from build123d import *

# Parameters (mm, degrees)
SKETCH2_R                = 6.25
BOSS_EXTRUDE1_DEPTH      = 24
BOSS_EXTRUDE1_DEPTH_BACK = 24
BOSS_EXTRUDE2_START      = 1
BOSS_EXTRUDE2_DEPTH      = 12.5
SKETCH5_R                = 5
BOSS_EXTRUDE4_DEPTH      = 10
BOSS_EXTRUDE4_DEPTH_BACK = 54
SKETCH6_R                = 6
BOSS_EXTRUDE5_DEPTH      = 31
BOSS_EXTRUDE5_DEPTH_BACK = 30


with BuildPart() as part:
    # Sketch2 → Boss-Extrude1 (new body, two sides)
    with BuildSketch(Plane(origin=(0, 0, 0), x_dir=(1, 0, 0), z_dir=(0, 1, 0))) as boss_extrude1_sk:
        with BuildLine():
            Line((270.578703704, 12.486596895), (1.157407407, 24.97319379))
            ThreePointArc((1.157407407, 24.97319379), (-25, 0), (1.157407407, -24.97319379))
            Line((1.157407407, -24.97319379), (270.578703704, -12.486596895))
            ThreePointArc((270.578703704, -12.486596895), (282.5, 0), (270.578703704, 12.486596895))
        make_face()
        Circle(SKETCH2_R, mode=Mode.SUBTRACT)
    extrude(amount=BOSS_EXTRUDE1_DEPTH)
    extrude(boss_extrude1_sk.sketch, amount=-BOSS_EXTRUDE1_DEPTH_BACK)



with BuildPart() as body_2:
    # Sketch3 → Boss-Extrude2 (new body)
    with BuildSketch(Plane(origin=(0, 24, 0), x_dir=(1, 0, 0), z_dir=(0, 1, 0)).offset(BOSS_EXTRUDE2_START)):
        with BuildLine():
            Line((270, 12.5), (350, 12.5))
            ThreePointArc((350, 12.5), (362.5, 0), (350, -12.5))
            Line((350, -12.5), (270, -12.5))
            ThreePointArc((270, -12.5), (257.5, 0), (270, 12.5))
        make_face()
    boss_extrude2 = extrude(amount=BOSS_EXTRUDE2_DEPTH)


with BuildPart() as part_1:
    add(part.part)

    add(body_2.part)  # Boss-Extrude4 merges body 2
    # Sketch5 → Boss-Extrude4 (add, two sides)
    with BuildSketch(Plane.XZ.offset(24)) as boss_extrude4_sk:
        with Locations((270, 0)):
            Circle(SKETCH5_R)
    extrude(amount=BOSS_EXTRUDE4_DEPTH)
    extrude(boss_extrude4_sk.sketch, amount=-BOSS_EXTRUDE4_DEPTH_BACK)

    # Mirror1: Boss-Extrude2 across plane
    add(boss_extrude2.mirror(Plane.ZX))

    # Sketch6 → Boss-Extrude5 (add, two sides)
    with BuildSketch(Plane(origin=(0, 0, 0), x_dir=(1, 0, 0), z_dir=(0, 1, 0))) as boss_extrude5_sk:
        with Locations((350, 0)):
            Circle(SKETCH6_R)
    extrude(amount=BOSS_EXTRUDE5_DEPTH)
    extrude(boss_extrude5_sk.sketch, amount=-BOSS_EXTRUDE5_DEPTH_BACK)


solid = part_1.part
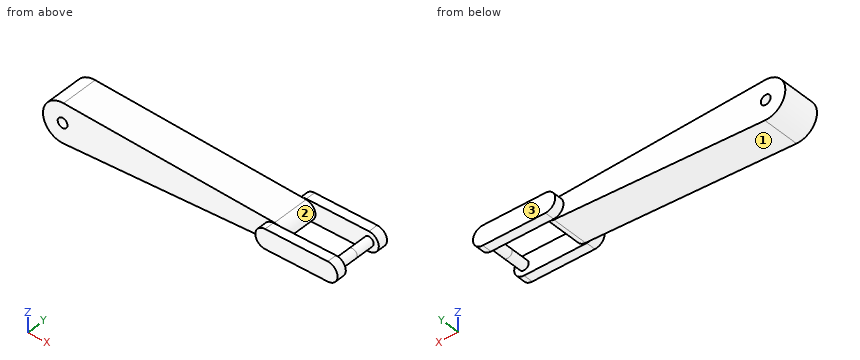
Source: CAD feature listing. Evaluate the final solid. Frame: model axes, mm. Face numbers are marked on the shaded views. Give positions to 0.01 mm unless a question says otherwise; leave off trailing zeros. Order: outer loops, then holes, each group sorted by start corner. A loop starts at its lowest first (then second) coordinate and runs counter-clockwise, first axis right, second up. Notation, with made-up numbers: (4.5, -15) -> (41.5, -15) arc R12 ccw to (41.5, -6) -> close; hole circle Ø3 at (46, 85.5). An arc over 180 degrees is marked (long way). Write item = value, one per line.
Item 1: Section query A-A (y = -10.5). Output: boundary loops of the cut face in (x, z), then the cut area to 3 significant figures.
Check result:
outline = (1.16, -24.97) -> (270.58, -12.49) arc R12.5 ccw to (270.58, 12.49) -> (1.16, 24.97) arc R25 ccw (long way) to start; circle Ø12 at (350, 0); hole circle Ø12.5 at (0, 0)
area = 11,400 mm²
Item 2: Ray query, probe 1 along Z at (x, y) = (0, 6); probe 2 along X at (y, z) = (-13.5, 4); probe 3 along Y at (x, z) = (340, 8.5). Return the intervals inside material, ascending.
Check result:
probe_1 = -25 to -6.25, 6.25 to 25
probe_2 = -24.68 to -4.8, 4.8 to 281.84, 345.53 to 354.47
probe_3 = -37.5 to -25, 25 to 37.5
Item 3: Section query C-C (z = 20). Output: boundary loops of the cut face in (x, y).
Check result:
outline = (-15, -24) -> (108.46, -24) -> (108.46, 24) -> (-15, 24) -> close
Item 4: Section query D-D (x = 244.5). Output: boundary loops of the cut face in (y, z), then the cut area to 3 significant figures.
Check result:
outline = (-24, -13.7) -> (24, -13.7) -> (24, 13.7) -> (-24, 13.7) -> close
area = 1,310 mm²
Item 5: Section query B-B (x = 322). Output: boundary loops of the cut face in (y, z), then the cut area to 3 significant figures.
Check result:
outline = (-37.5, -12.5) -> (-25, -12.5) -> (-25, 12.5) -> (-37.5, 12.5) -> close; (25, -12.5) -> (37.5, -12.5) -> (37.5, 12.5) -> (25, 12.5) -> close
area = 625 mm²
Item 6: Contact query for flat-ended pins moving along their axis: pin 1 (8 mm diameter, centred on x = 66, y = 20.5, fed in from -Z); pin 2 (5 mm diameter, centred on y = -5.5, z = -10.5, fed in from +X); pin 3 (12 mm diameter, centred on y = -8, z = -10, fed in from -X). Output: stop coordinate, or through.
Check result:
pin_1 = -22.15
pin_2 = 279.6
pin_3 = -24.68
Item 7: Mould query, pull axis X, two halves, no side actions, for the marked faces 1, 2 and 3. Classes: +X half, -X half, draft (parallel to the pull), parting line (faces both ways), or undercut.
Check result:
face_1 = +X half
face_2 = undercut
face_3 = draft
